Autodesk Inventor part; units mm, degrees
ref_plane "SHELL Plane" through (-494.9747, -494.9747, 0) normal (0.7071, -0.7071, 0) x (0.7071, 0.7071, 0)
ref_plane "ACCESS Plane" through (-265, -1100, 0) normal (0, -1, 0) x (1, 0, 0)
ref_plane "OUTER Plane" through (57, 900, 0) normal (0, 1, 0) x (-1, 0, 0)
sketch "floor angle sketch" plane through (0, 0, 0) normal (0, 0, 1) x (1, 0, 0)
  line L0 (0, 0) -> (0, -240.1382) construction
  line L1 (0, 0) -> (0, -1100)
  line L2 (-494.9747, -494.9747) -> (494.9747, 494.9747) construction
  circle A0 centre (0, 0) radius 700 construction
  line L3 (0, 0) -> (0, 900)
  line L4 (57, 900) -> (-57, 900)
  line L5 (-265, -1100) -> (265, -1100)
  line L6 (0, 0) -> (-342.0201, -939.6926)
  line L7 (0, 0) -> (0, 800)
  line L8 (57, 800) -> (-57, 800)
  line L9 (-403.1002, -917.4613) -> (-280.9401, -961.9239)
  dimension "d51" = 1400
  dimension "d52" = 45
  dimension "d54" = 0
  dimension "d55" = 180
  dimension "d56" = 530
  dimension "d58" = 114
  dimension "d59" = 114
  dimension "d60" = 180
  dimension "d61" = 800
  dimension "d62" = 130
  dimension "d63" = 20
  dimension "d64" = 900
  dimension "d65" = 1000
  dimension "d66" = 1100
ref_plane "SHELL Plane" through (-494.9747, -494.9747, 0) normal (0.7071, -0.7071, 0) x (0.7071, 0.7071, 0)
ref_plane "ACCESS Plane" through (-265, -1100, 0) normal (0, -1, 0) x (1, 0, 0)
ref_plane "OUTER Plane" through (57, 900, 0) normal (0, 1, 0) x (-1, 0, 0)
ref_plane "INNER Plane" through (57, 800, 0) normal (0, 1, 0) x (-1, 0, 0)
ref_plane "CHARGE Plane" through (-403.1002, -917.4613, 0) normal (-0.342, -0.9397, 0) x (0.9397, -0.342, 0)
sketch "Sketch13" plane through (-494.9747, -494.9747, 0) normal (0.7071, -0.7071, 0) x (0.7071, 0.7071, 0)
  line L0 (700, 0) -> (700, 892.6829)
  line L1 (0, 0) -> (6, 0)
  line L2 (6, 0) -> (6, 1400)
  line L3 (6, 1400) -> (0, 1400)
  line L4 (0, 1400) -> (0, 0)
  dimension "d75" = 1400
  dimension "d76" = 6
  dimension "d77" = 1400
revolve "Revolution2" add sketch "Sketch13" angle 359.9 about axis through (0, 0, 0) along (0, 0, 1)
sketch "Sketch14" plane through (-265, -1100, 0) normal (0, -1, 0) x (1, 0, 0)
  circle A0 centre (265, 1000) radius 265
  point P0 (265, 0)
  dimension "d79" = 1000
  dimension "d80" = 530
extrude "ACCESS" cut sketch "Sketch14" against normal up to next
sketch "Sketch15" plane through (57, 800, 0) normal (0, 1, 0) x (-1, 0, 0)
  circle A0 centre (57, 270) radius 58
  point P0 (57, 0)
  dimension "d84" = 116
  dimension "d85" = 270
extrude "INNER" cut sketch "Sketch15" against normal up to next
sketch "Sketch16" plane through (57, 900, 0) normal (0, 1, 0) x (-1, 0, 0)
  circle A0 centre (57, 1050) radius 58
  point P0 (57, 0)
  dimension "d88" = 1050
  dimension "d89" = 116
extrude "Extrusion9" cut sketch "Sketch16" against normal up to next
equation "\"BendRadius\" = Thickness"
equation "\"BendReliefWidth\" = Thickness"
equation "\"BendReliefDepth\" = 0.5 * Thickness"
equation "\"CornerReliefSize\" = 4 * Thickness"
equation "\"MinimumRemnant\" = 2 * Thickness"
equation "\"TransitionRadius\" = BendRadius"
equation "\"JacobiRadiusSize\" = BendRadius"
equation "\"GapSize\" = Thickness"
properties part number "ANP 1402 SHELL D1400" material "Steel"
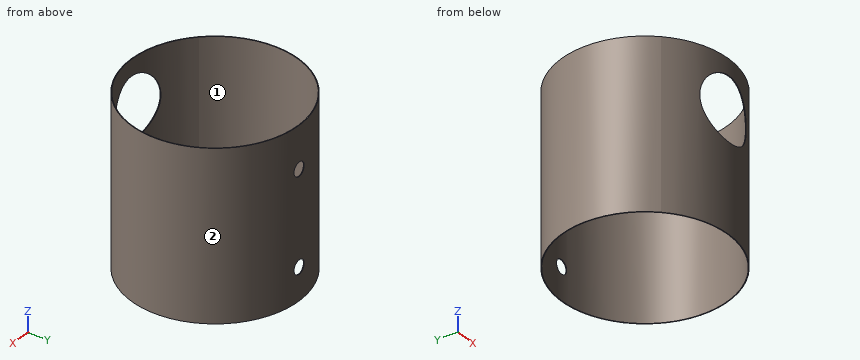
Model file for the job. Use its own axes, mm. Face numbers are marked on the shaded views. Give positions to 0.01 mm unless a question says otherwise; leave off trailing zeros. Loops run counter-clockwise (first coordinate to the right, second up) from the corner with the lowest first, then second, coordinate; pieces in that order, holes last. Notation, with made-up numbers: (85, -11) - (95, -11) arc R11 cw to (95, -3) - close; hole circle Ø9 at (-12, 10). An arc over 180 degrees is marked (long way). One line per item, written item: value. Start each with the question number.
1. Slice it at B-B (x = 0). List the corners of the cut face in (y, z), plus the area to 3 significant figures.
2. Slice it at D-D (x = 182). List the corners of the cut face in (y, z), plus the area to 3 significant figures.
3. Slice it at C-C (z = 270). List the corners of the cut face in (x, y), plus the area to 3 significant figures.
4. Slice it at A-A (y = 0). List the corners of the cut face in (x, z), plus the area to 3 significant figures.
5. Pull direction Y, two halves, no side cores. Call the marked faces 1 and 2: pulls with the +Y half, pulls with the -Y half, needs draft (parallel to the pull), parting line crosses it, or undercut.
6. Pin check, flat tips, straight feed: pin 1 (3 mm diameter, centred on x = 418.5, z = 967.5, fed in from +Y); pin 2 (8 mm diameter, centred on y = -168, z = 1142.5, fed in from +X); pin 3 (10 mm diameter, centred on x = 270, z = 428.5, fed in from -Y). Stop position of each tip, or through.
7. Probe L1, parallel to X at y = 0, z = 867.5; L2, parallel to X at y = -421, z = 383; L3, parallel to Y at x = 227, z = 611.5. List the from-to ranges inside material, lowest first. Write a range as from..to.
Solution:
1. outline: (-700, 0) - (-694, 0) - (-694, 735) - (-700, 735) - close; (-700, 1265) - (-694, 1265) - (-694, 1400) - (-700, 1400) - close; (694, 0) - (700, 0) - (700, 212) - (694, 212) - close; (694, 328) - (700, 328) - (700, 992) - (694, 992) - close; (694, 1108) - (700, 1108) - (700, 1400) - (694, 1400) - close
1. area: 12,200 mm^2
2. outline: (-675.93, 0) - (-669.71, 0) - (-669.71, 807.38) - (-675.93, 807.38) - close; (-675.93, 1192.62) - (-669.71, 1192.62) - (-669.71, 1400) - (-675.93, 1400) - close; (669.71, 0) - (675.93, 0) - (675.93, 1400) - (669.71, 1400) - close
2. area: 15,000 mm^2
3. outline: (-495.84, -494.11) - (-491.59, -489.87) arc R694 cw to (-58, 691.57) - (-58, 697.59) arc R700 ccw to start; (-494.97, -494.97) arc R700 ccw (long way) to (58, 697.59) - (58, 691.57) arc R694 cw (long way) to (-490.73, -490.73) - close
3. area: 25,600 mm^2
4. outline: (-700, 0) - (-694, 0) - (-694, 1400) - (-700, 1400) - close; (694, 0) - (700, 0) - (700, 1400) - (694, 1400) - close
4. area: 16,800 mm^2
5. face 1: undercut
5. face 2: parting line crosses it
6. pin 1: stops at y = 562.24
6. pin 2: stops at x = 680.52
6. pin 3: stops at y = -647.9
7. L1: x = -700..-694, 694..700
7. L2: x = -559.25..-551.72, 551.72..559.25
7. L3: y = -662.17..-655.83, 655.83..662.17
